```python
from build123d import *

# Parameters (mm, degrees)
SKETCH1_R           = 4
BOSS_EXTRUDE1_DEPTH = 21
SKETCH2_R           = 3.2
CUT_EXTRUDE1_DEPTH  = 10
SKETCH3_R           = 2.5
CUT_EXTRUDE3_DEPTH  = 10


with BuildPart() as part:
    # Sketch1 → Boss-Extrude1 (new body)
    with BuildSketch(Plane(origin=(0, 0, 0), x_dir=(1, 0, 0), z_dir=(0, 1, 0))):
        with Locations(Location((0, 0, 0), (0, 0, 90))):
            Circle(SKETCH1_R)
    extrude(amount=BOSS_EXTRUDE1_DEPTH)

    # Sketch2 → Cut-Extrude1 (cut)
    with BuildSketch(Plane.XZ):
        with Locations(Location((0, 0, 0), (0, 0, 270))):
            Circle(SKETCH2_R)
    extrude(amount=-CUT_EXTRUDE1_DEPTH, mode=Mode.SUBTRACT)

    # Sketch3 → Cut-Extrude3 (cut)
    with BuildSketch(Plane(origin=(0, 21, 0), x_dir=(1, 0, 0), z_dir=(0, 1, 0))):
        with Locations(Location((0, 0, 0), (0, 0, 270))):
            Circle(SKETCH3_R)
    extrude(amount=-CUT_EXTRUDE3_DEPTH, mode=Mode.SUBTRACT)

    # Cut-Extrude5: read off the stored shape, not the designer's step
    # Cut-Extrude5: loft between two sections, ruled curve by curve
    cut_extrude5_from = [
        Edge.make_three_point_arc((-2.07101841, 14.6, 0), (-2.07101841, 16, 1.4), (-2.07101841, 17.4, 0)),
        Edge.make_three_point_arc((-2.07101841, 17.4, 0), (-2.07101841, 16, -1.4), (-2.07101841, 14.6, 0)),
    ]
    cut_extrude5_to = [
        Edge.make_three_point_arc((-3.999916451, 14.6, 0), (-3.999916451, 16, 1.4), (-3.999916451, 17.4, 0)),
        Edge.make_three_point_arc((-3.999916451, 17.4, 0), (-3.999916451, 16, -1.4), (-3.999916451, 14.6, 0)),
    ]
    cut_extrude5 = Solid(Shell([*[Face.make_surface_from_curves(cut_extrude5_from[k], cut_extrude5_to[k]) for k in range(2)], Face(Wire(cut_extrude5_from)), Face(Wire(cut_extrude5_to))]))
    add(cut_extrude5, mode=Mode.SUBTRACT)

    # Cut-Extrude5 2: loft between two sections, ruled curve by curve
    cut_extrude5_2_from = [
        Edge.make_three_point_arc((-2.877351837, 3.6, 0), (-2.877351837, 5, 1.4), (-2.877351837, 6.4, 0)),
        Edge.make_three_point_arc((-2.877351837, 6.4, 0), (-2.877351837, 5, -1.4), (-2.877351837, 3.6, 0)),
    ]
    cut_extrude5_2_to = [
        Edge.make_three_point_arc((-3.999916451, 3.6, 0), (-3.999916451, 5, 1.4), (-3.999916451, 6.4, 0)),
        Edge.make_three_point_arc((-3.999916451, 6.4, 0), (-3.999916451, 5, -1.4), (-3.999916451, 3.6, 0)),
    ]
    cut_extrude5_2 = Solid(Shell([*[Face.make_surface_from_curves(cut_extrude5_2_from[k], cut_extrude5_2_to[k]) for k in range(2)], Face(Wire(cut_extrude5_2_from)), Face(Wire(cut_extrude5_2_to))]))
    add(cut_extrude5_2, mode=Mode.SUBTRACT)


solid = part.part
```
Source: CAD feature listing. Evaluate the final solid. Frame: model axes, mm. A direction names the side the tool comes from. Round coordinates to 2 decimals unless told otherwise and drop trailing zeros. Loops run counter-clockwise (first coordinate to the right, second up) from the corner with the lowest first, then second, coordinate; pieces in that order, holes last.
(1) Section query D-D (z = -0.5). Give the number of separate pieces and of enclosed holes in the cut face, and give its area (3 significant figures).
From the geometry:
separate pieces: 3
enclosed holes: 0
area: 48.4 mm2
(2) Section query C-C (z = 2.25). Output: boundary loops of the cut face in (x, y), and give its area (3 significant figures).
From the geometry:
outline: (-3.31, 0) - (-2.28, 0) - (-2.28, 10) - (2.28, 10) - (2.28, 0) - (3.31, 0) - (3.31, 21) - (1.09, 21) - (1.09, 11) - (-1.09, 11) - (-1.09, 21) - (-3.31, 21) - close
area: 71.6 mm2
(3) Material intervals for probe 1 along X at (y, z) = (14, 0); probe 2 along X at (y, z) = (7, 0); probe 3 along Y at (x, z) = (-1.75, 2.5), sorted ascending.
From the geometry:
probe 1: x = -4 to -2.5, 2.5 to 4
probe 2: x = -4 to -3.2, 3.2 to 4
probe 3: y = 10 to 21
(4) Section query A-A (x = 0). Output: boundary loops of the cut face in (y, z).
From the geometry:
outline: (0, -4) - (21, -4) - (21, -2.5) - (11, -2.5) - (11, 2.5) - (21, 2.5) - (21, 4) - (0, 4) - (0, 3.2) - (10, 3.2) - (10, -3.2) - (0, -3.2) - close
(5) Section query B-B (y = 14). Output: boundary loops of the cut face in (x, z), and give its area (3 significant figures).
From the geometry:
outline: circle Ø8 at (0, 0); hole circle Ø5 at (0, 0)
area: 30.6 mm2
(6) Pull-direction query (Z, two-part tool) for faces 4 (the flat face through (0, 10, 0)), 5 (the flat face through (-3, 0, 2)), 6 (the cylindrical face through (3.905, 10.353, 0.867)); classes: +Z half, -Z half, draft (parallel to the pull), parting line (faces both ways), or undercut.
From the geometry:
face 4: undercut
face 5: draft
face 6: parting line
(7) Contact query for flat-ended pins moving along their axis: pin 1 Ø2 at (x, y) = (2, 15.5) entering from -Z; pin 2 Ø3 at (x, z) = (2, 0) entering from -Y; pin 3 Ø2 at (y, z) = (3, -2.5) entering from -X; pin 4 Ø1 at (y, z) = (15, 1.5) entering from -X. Output: stop coordinate, or through.
From the geometry:
pin 1: stops at z = -3.87
pin 2: stops at y = 0
pin 3: stops at x = -3.71
pin 4: stops at x = -3.87
(8) Access query for faces 1 (the cylindrical face through (2.7, 4.93, -1.72)), 2 (the flat face through (-2, 21, -2)), 3 (the cylindrical face through (2.48, 16.07, -0.33)). Directions: +Z, -Z, +X, -X, +Y, -Y. A direction counts if a zero-diameter tool reaches every point of the face in a straight line with its end or side. Return the directions, or none.
From the geometry:
face 1: -Y
face 2: +Z, -Z, +X, -X, +Y
face 3: +Y
